Source: CAD feature listing. Evaluate the final solid. Frame: model axes, mm. A direction names the side the tool comes from. Coordinates: 2 decimals unless noted, no trailing zeros. Order: outer loops, then holes, each group sorted by start corner. A loop starts at its lowest first (then second) coordinate and runs counter-clockwise, first axis right, second up.
```python
from build123d import *

# Parameters (mm, degrees)
F1_DEPTH = 0.5
F3_DEPTH = 1.2
F4_R     = 0.75
F5_DEPTH = 2
F6_R     = 0.75
F7_DEPTH = 3.8
F8_SIZE  = 0.3
F9_SCALE = 3


with BuildPart() as f1:
    # F0 (on Top) → F1 (new body)
    with BuildSketch(Plane.XY):
        with BuildLine():
            Line((-0.2, -1.4866068747), (-0.2, 1.4866068747))
            ThreePointArc((-0.2, 1.4866068747), (-1.5, 0), (-0.2, -1.4866068747))
        make_face()
    extrude(amount=F1_DEPTH)



with BuildPart() as f1b:
    # F0 (on Top) → F1, piece 2 (new body)
    with BuildSketch(Plane.XY):
        with BuildLine():
            ThreePointArc((0.2, -1.4866068747), (1.5, 0), (0.2, 1.4866068747))
            Line((0.2, 1.4866068747), (0.2, -1.4866068747))
        make_face()
    extrude(amount=F1_DEPTH)


with BuildPart() as f1_1:
    add(f1.part)

    add(f1b.part)  # F3 merges F1b
    # F2 (on face) → F3 (join)
    with BuildSketch(Plane.XY.offset(0.5)):
        with BuildLine():
            Line((-0.2, -1.4866068747), (-0.2, 1.4866068747))
            ThreePointArc((-0.2, 1.4866068747), (-1.5, 0), (-0.2, -1.4866068747))
        make_face()
        with BuildLine():
            ThreePointArc((-0.2, -1.4866068747), (0.9874208829, -1.1291589791), (1.5, 0))
            ThreePointArc((1.5, 0), (0.9874208829, 1.1291589791), (-0.2, 1.4866068747))
            Line((-0.2, 1.4866068747), (-0.2, -1.4866068747))
        make_face()
    extrude(amount=F3_DEPTH)

    # F4 (on face) → F5 (join)
    with BuildSketch(Plane.XY.offset(1.7)):
        Circle(F4_R)
    extrude(amount=F5_DEPTH)

    # F6 (on face) → F7 (join)
    with BuildSketch(Plane.XY.offset(3.7)):
        Circle(F6_R)
    extrude(amount=F7_DEPTH)

    # F8
    f8_edges = [f1_1.edges().sort_by_distance(p)[0] for p in [
        (-0.75, 0, 7.5),
    ]]
    chamfer(f8_edges, length=F8_SIZE)


with BuildPart() as f1_2:
    # F9: moved
    add(f1_1.part.scale(F9_SCALE))


solid = f1_2.part
```
Q1. Section query B-B on z = 6.25. Output: boundary loops of the cut face in (x, y), plus the area to 3 significant figures.
Solutions:
outline: circle Ø4.5 at (0, 0)
area: 15.9 mm2
Q2. Section query A-A on x = 0. Output: boundary loops of the cut face in (y, z), plus the area to 3 significant figures.
Solutions:
outline: (-4.5, 1.5) - (4.5, 1.5) - (4.5, 5.1) - (2.25, 5.1) - (2.25, 21.6) - (1.35, 22.5) - (-1.35, 22.5) - (-2.25, 21.6) - (-2.25, 5.1) - (-4.5, 5.1) - close
area: 110 mm2
Q3. Pull-direction query (X, two-part tool) for faces 1 (the cylindrical face through (-0.29, 2.23, 13.23)), 2 (the flat face through (0.6, 0, 1)), 3 (the flat face through (2, 0, 0)); classes: pulls with the +X half, pulls with the -X half, needs draft (parallel to the pull), parting line crosses it, or undercut.
Solutions:
face 1: parting line crosses it
face 2: undercut
face 3: needs draft
Q4. Set-up query: faces 4 (the flat face through (2, -2, 5.1)), 5 (the flat face through (0, 0, 1.5)), 6 (the flat face through (0, 0, 22.5)). Return all of +Z, -Z, +X, -X, +Y, -Y with unobstructed straight access to the full face (end or side cutting, diameter ignored); none if empty.
Solutions:
face 4: +Z
face 5: -Z, +Y, -Y
face 6: +Z, +X, -X, +Y, -Y
Q5. Pin query (flat end, axial travel): P1, Ø4, axis at x = 1, y = -1, coming from the +Z side; P2, Ø2, axis at x = 2, y = 1.5, coming from the +Z side; P3, Ø2, axis at y = -3, z = 5.5, coming from the +X side; P4, Ø1.5, axis at x = 0, z = 12, coming from the +Y side. Return the tip coordinate at first contact, or that it passes through.
Solutions:
P1: stops at z = 22.5
P2: stops at z = 22.35
P3: stops at x = 3.99
P4: stops at y = 2.25
Q6. Material intervals for line 1 along Z through (x, y) = (-2, -2.25); line 2 along Z through (x, y) = (-0.5, -3.5); line 3 along Y through (x, z) = (0.25, 21), sorted ascending.
Solutions:
line 1: z = 0 to 5.1
line 2: z = 1.5 to 5.1
line 3: y = -2.24 to 2.24
Q7. Section query D-D on x = -4. Output: boundary loops of the cut face in (y, z).
Solutions:
outline: (-2.06, 0) - (2.06, 0) - (2.06, 5.1) - (-2.06, 5.1) - close
Q8. Section query C-C on y = 3.25. Output: boundary loops of the cut face in (x, z), plus the area to 3 significant figures.
Solutions:
outline: (-3.11, 0) - (-0.6, 0) - (-0.6, 1.5) - (0.6, 1.5) - (0.6, 0) - (3.11, 0) - (3.11, 5.1) - (-3.11, 5.1) - close
area: 29.9 mm2
